from build123d import *

# Parameters (mm, degrees)
CYLINDER002_R     = 2
CYLINDER002_DEPTH = 2
ARRAY001_X_COUNT  = 2
ARRAY001_X_PITCH  = 28
ARRAY001_Y_COUNT  = 2
ARRAY001_Y_PITCH  = 28
CYLINDER001_R     = 1
CYLINDER001_DEPTH = 10
ARRAY_X_COUNT     = 2
ARRAY_X_PITCH     = 28
ARRAY_Y_COUNT     = 2
ARRAY_Y_PITCH     = 28
BOX_W             = 40
BOX_H             = 40
BOX_DEPTH         = 5
FILLET_R          = 3
FILLET001_R       = 2


with BuildPart() as array001:
    # Cylinder002 → Cylinder002 (new body)
    with BuildSketch(Plane(origin=(6, 6, 3), x_dir=(1, 0, 0), z_dir=(0, 0, 1))):
        Circle(CYLINDER002_R)
    extrude(amount=CYLINDER002_DEPTH)

    # Array001 X: Array001 ×2


with BuildPart() as array001_1:
    add(array001.part)
    with Locations(*[(i * ARRAY001_X_PITCH, 0, 0) for i in range(1, ARRAY001_X_COUNT)]):
        add(array001.part)

    # Array001 Y: Array001 ×2


with BuildPart() as array001_2:
    add(array001_1.part)
    with Locations(*[(0, i * ARRAY001_Y_PITCH, 0) for i in range(1, ARRAY001_Y_COUNT)]):
        add(array001_1.part)


with BuildPart() as array:
    # Cylinder001 → Cylinder001 (new body)
    with BuildSketch(Plane(origin=(6, 6, -2), x_dir=(1, 0, 0), z_dir=(0, 0, 1))):
        Circle(CYLINDER001_R)
    extrude(amount=CYLINDER001_DEPTH)

    # Array X: Array ×2


with BuildPart() as array_1:
    add(array.part)
    with Locations(*[(i * ARRAY_X_PITCH, 0, 0) for i in range(1, ARRAY_X_COUNT)]):
        add(array.part)

    # Array Y: Array ×2


with BuildPart() as array_2:
    add(array_1.part)
    with Locations(*[(0, i * ARRAY_Y_PITCH, 0) for i in range(1, ARRAY_Y_COUNT)]):
        add(array_1.part)


with BuildPart() as cut002:
    # Box → Box (new body)
    with BuildSketch(Plane.XY):
        with Locations((20, 20)):
            Rectangle(BOX_W, BOX_H)
    extrude(amount=BOX_DEPTH)

    # Fillet
    fillet_edges = [cut002.edges().sort_by_distance(p)[0] for p in [
        (0, 0, 2.5),
        (0, 40, 2.5),
        (40, 0, 2.5),
        (40, 40, 2.5),
    ]]
    fillet(fillet_edges, radius=FILLET_R)

    # Fillet001
    fillet001_edges = [cut002.edges().sort_by_distance(p)[0] for p in [
        (0, 20, 5),
        (0.87868, 0.87868, 5),
        (0.87868, 39.12132, 5),
        (20, 0, 5),
        (20, 40, 5),
        (39.12132, 0.87868, 5),
        (39.12132, 39.12132, 5),
        (40, 20, 5),
    ]]
    fillet(fillet001_edges, radius=FILLET001_R)

    # Cut001: cut Array
    add(array_2.part, mode=Mode.SUBTRACT)

    # Cut002: cut Array001
    add(array001_2.part, mode=Mode.SUBTRACT)


solid = cut002.part
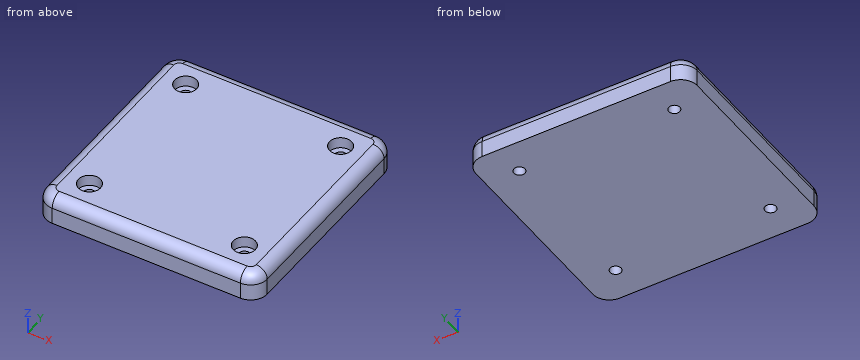
Work out the finished part from the listing and answer in its coordinate system (mm). Give positions to 0.01 mm unless a question says otherwise; leave off trailing zeros. Loops run counter-clockwise (first coordinate to the right, second up) from the corner with the lowest first, then second, coordinate; pieces in that order, holes last. Notation, with made-up numbers: (73, 38.25) -> (87, 38.25) arc R10 ccw to (87, 48.25) -> close; hole circle Ø6 at (27, 14). An arc over 180 degrees is marked (long way). Use a Markdown table: item, result. Add a question column.
1) The part is cut by section C-C, the plane z = 4.15. Count the separate pieces of the cut face and the enclosed holes in it, plus the area to 3 significant figures.
2) The part is cut by section A-A, the plane y = 6. Determine the outline of the cut face in (x, z), plus the area to 3 significant figures.
3) This flat-tipped pin is pushed along its axis until it touches: P1, Ø2.5, axis at x = 6, y = 34, coming from the +Z side. Where does it stop, or does it pass through?
4) Consider line 1 along X through (y, z) = (6, 1.8); line 2 along Y through (x, z) = (6, 3.8). Determine where each line is inside the solid, lowest interval first.
Reported:
| question | item | result |
|---|---|---|
| 1 | separate pieces | 1 |
| 1 | enclosed holes | 4 |
| 1 | area | 1,490 mm^2 |
| 2 | outline | (0, 0) -> (5, 0) -> (5, 3) -> (4, 3) -> (4, 5) -> (2, 5) arc R2 ccw to (0, 3) -> close; (7, 0) -> (33, 0) -> (33, 3) -> (32, 3) -> (32, 5) -> (8, 5) -> (8, 3) -> (7, 3) -> close; (35, 0) -> (40, 0) -> (40, 3) arc R2 ccw to (38, 5) -> (36, 5) -> (36, 3) -> (35, 3) -> close |
| 2 | area | 170 mm^2 |
| 3 | P1 | stops at z = 3 |
| 4 | line 1 | x = 0 to 5, 7 to 33, 35 to 40 |
| 4 | line 2 | y = 0.17 to 4, 8 to 32, 36 to 39.83 |
